Check sheet for the modelled part. Datum: model origin and axes. Units: mm. Face numbers are marked on the shaded views. A direction names the side the tool comes from. Round coordinates to 2 decimals unless told otherwise and drop trailing zeros. Order: outer loops, then holes, each group sorted by start corner. A loop starts at its lowest first (then second) coordinate and runs counter-clockwise, first axis right, second up. Notation, with made-up numbers: (8.25, 85) -> (19.25, 85) arc R4 ccw to (19.25, 92) -> close; hole circle Ø1 at (25, 75.25). An arc over 180 degrees is marked (long way). Answer in a Markdown table with one row per item. Add a question column.
1. Material ranges on L1, parallel to X at y = 8.6, z = -6; L2, parallel to Y at x = 10, z = -3.75, recorded low to high. Write a range as from..to.
2. Sectioned sample at A-A, the plane x = 13.75. Record the boundary of the cut face in (y, z), then the cut area to 3 significant figures.
3. Depth check by flat-ended pin: P1, Ø2.5, axis at x = 13.75, z = -6, coming from the -Y side; P2, Ø1.8, axis at x = -9.5, z = -10, coming from the +Y side; P3, Ø3.5, axis at y = -6.5, z = -4.5, coming from the +X side; P4, Ø1.2, axis at x = -13.75, z = -6, coming from the -Y side. Enter the tip coordinate at first touch or a pass-through.
4. Sectioned sample at C-C, the plane x = 1. Record the boundary of the cut face in (y, z).
5. Sectioned sample at D-D, the plane z = -2. Record the boundary of the cut face in (x, y).
6. Access from +Z, -Z, +X, -X, +Y, -Y to the whole of each face (thin tool, end or side, straight path). Record for the marked faces 1, 2, 3 and 4.
7. Sectioned sample at B-B, the plane y = 8. Record the boundary of the cut face in (x, z).
```python
from build123d import *

# Parameters (mm, degrees)
SKETCH_1_W                      = 22.5
SKETCH_1_H                      = 22.5
EXTRUDE_1_DEPTH                 = 12
SKETCH_2_W                      = 12
SKETCH_2_H                      = 2.7
EXTRUDE_2_DEPTH                 = 5
CUT_EXTRUDE_1_REACH             = 30.78
SKETCH_4_R                      = 1
CUT_EXTRUDE_1_DIRECTION_2_DEPTH = 29.78041869
EXTRUDE_3_DEPTH                 = 6
SKETCH_6_R                      = 2.4
EXTRUDE_4_DEPTH                 = 3.8


with BuildPart() as part:
    # 草图1 → 凸台-拉伸1 (new body)
    with BuildSketch(Plane.XY):
        Rectangle(SKETCH_1_W, SKETCH_1_H)
    extrude(amount=-EXTRUDE_1_DEPTH)

    # 草图2 → 凸台-拉伸2 (add)
    with BuildSketch(Plane(origin=(11.25, 0, 0), x_dir=(0, 0, -1), z_dir=(1, 0, 0))):
        with Locations((6, 7.9)):
            Rectangle(SKETCH_2_W, SKETCH_2_H)
    extrude(amount=EXTRUDE_2_DEPTH)

    # 草图4 → 切除-拉伸1 (cut, up to next)
    with BuildSketch(Plane(origin=(0, 9.25, 0), x_dir=(1, 0, 0), z_dir=(0, 1, 0)), mode=Mode.PRIVATE) as cut_extrude_1_sk1:
        with Locations(Location((13.75, 6, 0), (0, 0, 90))):
            Circle(SKETCH_4_R)
    cut_extrude_1_tool1 = extrude(cut_extrude_1_sk1.sketch, amount=-CUT_EXTRUDE_1_REACH, mode=Mode.PRIVATE) & part.part
    add(cut_extrude_1_tool1.solids().sort_by_distance((13.75, 9.25, -6))[0], mode=Mode.SUBTRACT)

    # 草图4 → 切除-拉伸1 direction 2 (cut)
    with BuildSketch(Plane(origin=(0, 9.25, 0), x_dir=(1, 0, 0), z_dir=(0, 1, 0))):
        with Locations(Location((13.75, 6, 0), (0, 0, 90))):
            Circle(SKETCH_4_R)
    extrude(amount=CUT_EXTRUDE_1_DIRECTION_2_DEPTH, mode=Mode.SUBTRACT)

    # 镜向1: part across plane


with BuildPart() as part_1:
    add(part.part)
    add(part.part.mirror(Plane(origin=(0, 0, 0), x_dir=(0, 0, 1), z_dir=(1, 0, 0))))

    # 草图5 → 凸台-拉伸3 (add)
    with BuildSketch(Plane(origin=(0, 11.25, 0), x_dir=(1, 0, 0), z_dir=(0, 1, 0))):
        with BuildLine():
            ThreePointArc((0.15, 8.615339366), (-11.25, 6), (0.15, 3.384660634))
            ThreePointArc((0.15, 3.384660634), (3.75, 6), (0.15, 8.615339366))
        make_face()
    extrude(amount=EXTRUDE_3_DEPTH)

    # 草图6 → 凸台-拉伸4 (add)
    with BuildSketch(Plane(origin=(0, 17.25, 0), x_dir=(1, 0, 0), z_dir=(0, 1, 0))):
        with Locations((-5.25, 6)):
            Circle(SKETCH_6_R)
    extrude(amount=EXTRUDE_4_DEPTH)


solid = part_1.part
```
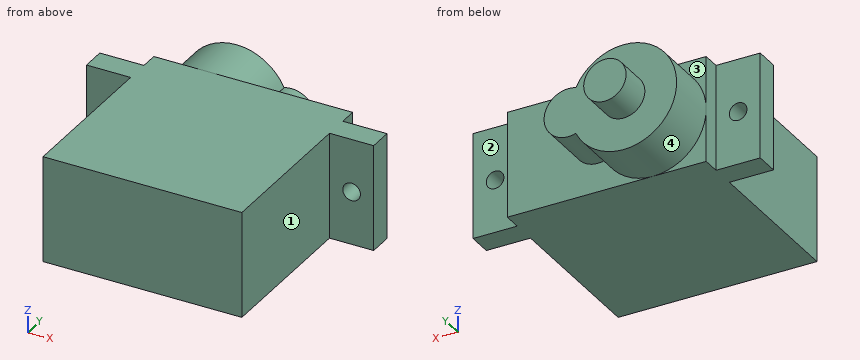
Answer key:
| question | item | result |
|---|---|---|
| 1 | L1 | x = -16.25..-14.75, -12.75..12.75, 14.75..16.25 |
| 1 | L2 | y = -11.25..11.25 |
| 2 | outline | (6.55, -12) -> (9.25, -12) -> (9.25, -7) -> (6.55, -7) -> close; (6.55, -5) -> (9.25, -5) -> (9.25, 0) -> (6.55, 0) -> close |
| 2 | area | 27.0 mm² |
| 3 | P1 | stops at y = 6.55 |
| 3 | P2 | stops at y = 17.25 |
| 3 | P3 | stops at x = 11.25 |
| 3 | P4 | passes through |
| 4 | outline | (-11.25, -12) -> (11.25, -12) -> (11.25, -8.75) -> (17.25, -8.75) -> (17.25, -3.25) -> (11.25, -3.25) -> (11.25, 0) -> (-11.25, 0) -> close |
| 5 | outline | (-16.25, 6.55) -> (-11.25, 6.55) -> (-11.25, -11.25) -> (11.25, -11.25) -> (11.25, 6.55) -> (16.25, 6.55) -> (16.25, 9.25) -> (11.25, 9.25) -> (11.25, 11.25) -> (-0.78, 11.25) -> (-0.78, 17.25) -> (-9.72, 17.25) -> (-9.72, 11.25) -> (-11.25, 11.25) -> (-11.25, 9.25) -> (-16.25, 9.25) -> close |
| 6 | face 1 | +Z, -Z, +X, -Y |
| 6 | face 2 | +Z, -Z, +X, +Y |
| 6 | face 3 | +Z, -X, +Y |
| 6 | face 4 | +Y |
| 7 | outline | (-16.25, -12) -> (16.25, -12) -> (16.25, 0) -> (-16.25, 0) -> close; hole circle Ø2 at (-13.75, -6); hole circle Ø2 at (13.75, -6) |
